from build123d import *

# Parameters (mm, degrees)
BOSS_EXTRUDE1_DEPTH = 12.7
BOSS_EXTRUDE2_DEPTH = 127
FILLET1_R           = 25.4
FILLET2_R           = 25.4
SKETCH1_5_W         = 80.645440106
SKETCH1_5_H         = 22.674837422
SKETCH1_5_W_2       = 79.142645348
BOSS_EXTRUDE3_DEPTH = 101.6
BOSS_EXTRUDE4_DEPTH = 12.7
BOSS_EXTRUDE5_DEPTH = 12.7
SKETCH5_R           = 12.7
BOSS_EXTRUDE7_DEPTH = 584.2
SKETCH7_W           = 228.6
SKETCH7_H           = 7.952880345
BOSS_EXTRUDE8_DEPTH = 8.636
SKETCH8_W           = 6.162041428
SKETCH8_H           = 183.673914537
BOSS_EXTRUDE9_DEPTH = 18.542


with BuildPart() as part:
    # Sketch1 → Boss-Extrude1 (new body)
    with BuildSketch(Plane(origin=(0, 0, 0), x_dir=(1, 0, 0), z_dir=(0, 1, 0))):
        Polygon((79.142645348, 22.674837422), (79.142645348, 0), (194.415916135, 0), (194.415916135, 22.674837422), (275.061356241, 22.674837422), (275.061356241, 0), (293.021868483, 17.960512242), (293.021868483, 22.674837422), (577.865587161, 22.674837422), (577.865587161, 114.3), (577.865587161, 205.925162578), (293.021868483, 205.925162578), (293.021868483, 210.639487758), (275.061356241, 228.6), (275.061356241, 205.925162578), (194.415916135, 205.925162578), (194.415916135, 228.6), (79.142645348, 228.6), (79.142645348, 205.925162578), (0, 205.925162578), (0, 22.674837422), align=None)
    extrude(amount=BOSS_EXTRUDE1_DEPTH)

    # Sketch1<4> → Boss-Extrude2 (add)
    with BuildSketch(Plane(origin=(0, 0, 0), x_dir=(1, 0, 0), z_dir=(0, 1, 0))):
        Polygon((577.865587161, 22.674837422), (577.865587161, 17.960512242), (586.043736966, 17.960512242), (586.043736966, 22.674837422), (586.043736966, 114.3), (586.043736966, 205.925162578), (586.043736966, 210.639487758), (577.865587161, 210.639487758), (577.865587161, 205.925162578), (577.865587161, 114.3), align=None)
    extrude(amount=BOSS_EXTRUDE2_DEPTH)

    # Fillet1
    fillet1_edges = [part.edges().sort_by_distance(p)[0] for p in [
        (581.954662063, 127, -17.960512242),
    ]]
    fillet(fillet1_edges, radius=FILLET1_R)

    # Fillet2
    fillet2_edges = [part.edges().sort_by_distance(p)[0] for p in [
        (581.954662063, 127, -210.639487758),
    ]]
    fillet(fillet2_edges, radius=FILLET2_R)

    # Sketch1<5> → Boss-Extrude3 (add)
    with BuildSketch(Plane(origin=(0, 0, 0), x_dir=(1, 0, 0), z_dir=(0, 1, 0))):
        with Locations((234.738636188, 217.262581289)):
            Rectangle(SKETCH1_5_W, SKETCH1_5_H)
        with Locations((39.571322674, 217.262581289)):
            Rectangle(SKETCH1_5_W_2, SKETCH1_5_H)
        with Locations((234.738636188, 11.337418711)):
            Rectangle(SKETCH1_5_W, SKETCH1_5_H)
        with Locations((39.571322674, 11.337418711)):
            Rectangle(SKETCH1_5_W_2, SKETCH1_5_H)
    extrude(amount=BOSS_EXTRUDE3_DEPTH)

    # Sketch2 → Boss-Extrude4 (add)
    with BuildSketch(Plane.XZ):
        Polygon((275.061356241, 0), (373.832124936, -98.770768695), (373.832124936, -129.829231305), (275.061356241, -228.6), (0, -228.6), (0, 0), align=None)
    extrude(amount=BOSS_EXTRUDE4_DEPTH)

    # Sketch4 → Boss-Extrude5 (add)
    with BuildSketch(Plane(origin=(0, 101.6, 0), x_dir=(1, 0, 0), z_dir=(0, 1, 0))):
        Polygon((275.061356241, 228.6), (297.736193663, 205.925162578), (297.736193663, 22.674837422), (275.061356241, 0), (0, 0), (0, 228.6), align=None)
    extrude(amount=BOSS_EXTRUDE5_DEPTH)

    # Sketch5 → Boss-Extrude7 (add)
    with BuildSketch(Plane(origin=(586.043736966, 0, 0), x_dir=(0, 0, -1), z_dir=(1, 0, 0))):
        with Locations((78.830256121, 114.3)):
            Circle(SKETCH5_R)
        with Locations((149.769743879, 114.3)):
            Circle(SKETCH5_R)
    extrude(amount=-BOSS_EXTRUDE7_DEPTH)

    # Sketch7 → Boss-Extrude8 (add)
    with BuildSketch(Plane.ZY):
        with Locations((-114.3, 110.323559828)):
            Rectangle(SKETCH7_W, SKETCH7_H)
    extrude(amount=BOSS_EXTRUDE8_DEPTH)

    # Sketch8 → Boss-Extrude9 (add)
    with BuildSketch(Plane(origin=(0, 114.3, 0), x_dir=(1, 0, 0), z_dir=(0, 1, 0))):
        with Locations((-5.554979286, 114.511794691)):
            Rectangle(SKETCH8_W, SKETCH8_H)
    extrude(amount=BOSS_EXTRUDE9_DEPTH)


solid = part.part
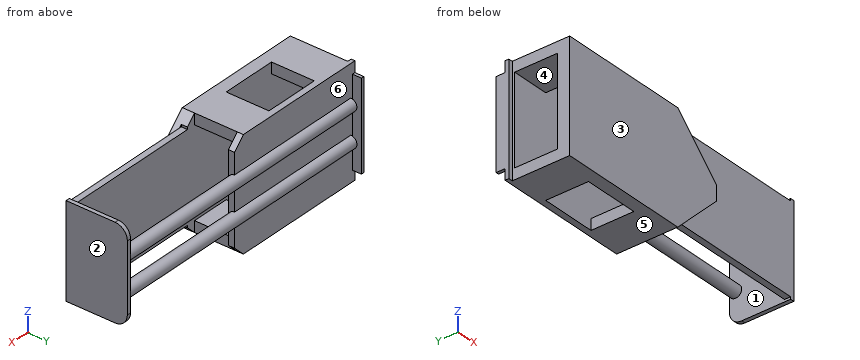
Source: CAD feature listing. Evaluate the final solid. Frame: model axes, mm. Face numbers are marked on the shaded views. A direction names the side the tool comes from. Round coordinates to 2 decimals unless told otherwise and drop trailing zeros. Loops run counter-clockwise (first coordinate to the right, second up) from the corner with the lowest first, then second, coordinate; pieces in that order, holes last.
Q1. Ray query, line 1 (Y direction, x = 257, z = -94.5); line 2 (Y direction, x = 102.5, z = -79); line 3 (Z direction, x = 235.5, y = 37). Return the intervals inside material, ascending.
Q2. Section D-D, the plane x = 138.5. Return loops of the section in (y, z).
Q3. Mould query, pull axis Z, two halves, no side actions, for the marked faces 3, 4, 5 and 6. Classes: pulls with the +Z half, pulls with the -Z half, needs draft (parallel to the pull), parting line crosses it, or undercut.
Q4. Access query for the marked faces 1 and 2. Directions: +Z, -Z, +X, -X, +Y, -Y. A direction counts if a zero-diameter tool reaches every point of the face in a straight line with its end or side. Return the directions, or none.
Q5. Section B-B, the plane z = -32. Return loops of the section in (x, y).
Q6. Section C-C, the plane x = 206. Return loops of the section in (y, z), plus the area to 3 significant figures.
Q7. First-contact query: P1, Ø2.5, axis at x = 582, y = 38, coming from the -Z side; P2, Ø25, axis at y = 36, z = -9, coming from the -X side; P3, Ø6.5, axis at x = 476, y = 5.5, coming from the -Z side; P4, Ø25, axis at y = 55, z = -16, coming from the +X side. Flat tips, straight axial feed; report the tip coordinate or a pass-through.
Q8. Section A-A, the plane y = 87.5. Return loops of the section in (x, z).
Solutions:
1. line 1: y = -12.7 to 12.7, 101.6 to 114.3
1. line 2: y = -12.7 to 12.7, 101.6 to 127
1. line 3: z = -228.6 to -205.93, -22.67 to 0
2. outline: (-12.7, -228.6) - (12.7, -228.6) - (12.7, 0) - (-12.7, 0) - close; (101.6, -228.6) - (114.3, -228.6) - (114.3, -162.47) arc R12.7 ccw to (114.3, -137.07) - (114.3, -91.53) arc R12.7 ccw to (114.3, -66.13) - (114.3, 0) - (101.6, 0) - close
3. face 3: needs draft
3. face 4: undercut
3. face 5: pulls with the -Z half
3. face 6: undercut
4. face 1: none
4. face 2: +Z, -Z, +X, +Y, -Y
5. outline: (-8.64, 106.35) - (0, 106.35) - (0, 101.6) - (297.74, 101.6) - (297.74, 114.3) - (-2.47, 114.3) - (-2.47, 132.84) - (-8.64, 132.84) - close; (0, -12.7) - (307.06, -12.7) - (307.06, 0) - (586.04, 0) - (586.04, 124.32) - (577.87, 124.32) - (577.87, 12.7) - (0, 12.7) - close
6. outline: (-12.7, -228.6) - (114.3, -228.6) - (114.3, -162.47) arc R12.7 ccw to (114.3, -137.07) - (114.3, -91.53) arc R12.7 ccw to (114.3, -66.13) - (114.3, 0) - (-12.7, 0) - close; hole (12.7, -205.93) - (101.6, -205.93) - (101.6, -22.67) - (12.7, -22.67) - close
6. area: 13,200 mm2
7. P1: stops at z = -210.64
7. P2: stops at x = 0
7. P3: stops at z = -205.93
7. P4: stops at x = 586.04
8. outline: (0, -228.6) - (79.14, -228.6) - (79.14, -205.93) - (0, -205.93) - close; (0, -22.67) - (79.14, -22.67) - (79.14, 0) - (0, 0) - close; (194.42, -228.6) - (275.06, -228.6) - (275.06, -205.93) - (194.42, -205.93) - close; (194.42, -22.67) - (275.06, -22.67) - (275.06, 0) - (194.42, 0) - close; (577.87, -210.64) - (586.04, -210.64) - (586.04, -17.96) - (577.87, -17.96) - close
